from build123d import *

# Parameters (mm, degrees)
SKETCH1_R           = 1.651
BOSS_EXTRUDE1_DEPTH = 1.5875
FILLET1_R           = 1.5875
FILLET2_R           = 0.396875
FILLET3_R           = 1.5875


with BuildPart() as part:
    # Sketch1 → Boss-Extrude1 (new body)
    with BuildSketch(Plane.XY):
        with BuildLine():
            Line((1.05664, 3.989958416), (1.05664, 9.8425))
            Line((1.05664, 9.8425), (0, 11.43))
            Line((0, 11.43), (-1.05664, 9.8425))
            Line((-1.05664, 9.8425), (-1.05664, 3.989958416))
            ThreePointArc((-1.05664, 3.989958416), (0, -4.1275), (1.05664, 3.989958416))
        make_face()
        Circle(SKETCH1_R, mode=Mode.SUBTRACT)
    extrude(amount=BOSS_EXTRUDE1_DEPTH)

    # Fillet1
    fillet1_edges = [part.edges().sort_by_distance(p)[0] for p in [
        (1.05664, 9.8425, 0.79375),
        (-1.05664, 9.8425, 0.79375),
    ]]
    fillet(fillet1_edges, radius=FILLET1_R)

    # Fillet2
    fillet2_edges = [part.edges().sort_by_distance(p)[0] for p in [
        (0, 11.43, 0.79375),
    ]]
    fillet(fillet2_edges, radius=FILLET2_R)

    # Fillet3
    fillet3_edges = [part.edges().sort_by_distance(p)[0] for p in [
        (1.05664, 3.989958416, 0.79375),
        (-1.05664, 3.989958416, 0.79375),
    ]]
    fillet(fillet3_edges, radius=FILLET3_R)


solid = part.part
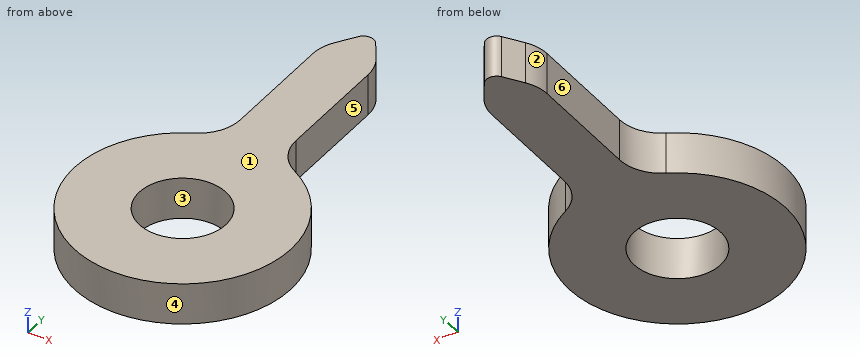
Work out the finished part from the listing and answer in its coordinate system (mm). Face numbers are marked on the shaded views. A direction names the side the tool comes from. Coordinates: 2 decimals unless noted, no trailing zeros. Order: outer loops, then holes, each group sorted by start corner. A loop starts at its lowest first (then second) coordinate and runs counter-clockwise, first axis right, second up. Notation, with made-up numbers: (55.25, 33.5) - (93.25, 33.5) arc R26 ccw to (93.25, 72.5) - close; hole circle Ø8 at (-36.75, -15.5). An arc over 180 degrees is marked (long way). Put each result on its own line as item: value. Start each with the question number.
1) Find section A-A (y = 0). Give the vertices of the cut face in (x, z), plus the area to 3 significant figures.
2) Flat-ended cylindrical pins translate along their axes: pin 1 (0.8 mm diameter, centred on y = 6, z = 1, fed in from +X); pin 2 (1 mm diameter, centred on x = -2, y = 5, fed in from -Z). Find the tip coordinate at first contact, or state that the pin passes through.
3) For a pull along Y with two mould halves and no side action, classify the marked faces 1, 2 and 3 as released by +Y, released by -Y, zero draft, split by the parting line, or undercut.
4) Find the intervals of material crossed by line 1 (X direction, y = 5.75, z = 0.75); line 2 (Y direction, x = 1.5, z = 1.25); line 3 (Y direction, x = -0.5, z = 1), in increasing order. Write a range as from..to.
5) Find section B-B (z = 1). Give the vertices of the cut face in (x, y) (1 decimal), plus the area to 3 significant figures.
6) Find section C-C (x = 0). Give the vertices of the cut face in (y, z).
7) For the marked faces 4, 5 and 6, determine the directions among +Z, -Z, +X, -X, +Y, -Y from which every point of the face is accessible in a straight line to the end or side of a thin tool.
8) Find section D-D (y = 6.25). Give the vertices of the cut face in (x, z), plus the area to 3 significant figures.
Results list:
1. outline: (-4.13, 0) - (-1.65, 0) - (-1.65, 1.59) - (-4.13, 1.59) - close; (1.65, 0) - (4.13, 0) - (4.13, 1.59) - (1.65, 1.59) - close
1. area: 7.86 mm^2
2. pin 1: stops at x = 1.06
2. pin 2: passes through
3. face 1: zero draft
3. face 2: released by +Y
3. face 3: undercut
4. line 1: x = -1.06..1.06
4. line 2: y = -3.85..-0.69, 0.69..3.97
4. line 3: y = -4.1..-1.57, 1.57..10.68
5. outline: (-1.9, 3.7) arc R4.1 ccw (long way) to (1.9, 3.7) arc R1.6 cw to (1.1, 5.1) - (1.1, 9.4) arc R1.6 ccw to (0.8, 10.2) - (0.3, 10.9) arc R0.4 ccw to (-0.3, 10.9) - (-0.8, 10.2) arc R1.6 ccw to (-1.1, 9.4) - (-1.1, 5.1) arc R1.6 cw to start; hole circle Ø3.3 at (0, 0)
5. area: 59.1 mm^2
6. outline: (-4.13, 0) - (-1.65, 0) - (-1.65, 1.59) - (-4.13, 1.59) - close; (1.65, 0) - (11.11, 0) - (11.11, 1.59) - (1.65, 1.59) - close
7. face 4: +Z, -Z
7. face 5: +Z, -Z, +X, +Y
7. face 6: +Z, -Z, -X, +Y
8. outline: (-1.06, 0) - (1.06, 0) - (1.06, 1.59) - (-1.06, 1.59) - close
8. area: 3.35 mm^2
